Autodesk Inventor part; units mm, degrees
ref_plane "Work Plane1" through (29, 0, 0) normal (0, -1, 0) x (1, 0, 0)
ref_plane "YZ Plane" through (0, 0, 0) normal (1, 0, 0) x (0, 1, 0)
ref_plane "XZ Plane" through (0, 0, 0) normal (0, 1, 0) x (-1, 0, 0)
sketch "Sketch1" plane through (0, 0, 0) normal (0, 0, 1) x (1, 0, 0)
  line L0 (-0.0762, 0) -> (3.175, 0)
  line L1 (3.175, 0) -> (3.175, 1.7526)
  line L2 (3.175, 1.7526) -> (1.5902, 1.7526)
  line L3 (1.5902, 1.7526) -> (0.0001, 1.7526)
  line L4 (0.0001, 1.7526) -> (0, 1.7526)
  line L5 (0, 1.7526) -> (0, 3.3274)
  line L6 (0, 3.3274) -> (-1.8542, 3.3274)
  line L7 (-1.8542, 3.3274) -> (-1.8542, 1.1438)
  line L8 (-1.8542, 1.1438) -> (-0.7366, 1.1438)
  line L9 (-0.7366, 1.1438) -> (-0.0762, 0)
  line L10 (-2.86, 0) -> (4.1808, 0)
  line L11 (0, -0.6655) -> (0, 3.9929)
  line L12 (1.5902, 1.7526) -> (0, 1.7526) construction
  dimension "d1" = 1.5848
  dimension "d2" = 1.5901
  dimension "d3" = 1.8542
  dimension "d4" = 1.1176
  dimension "d5" = 60
  dimension "d6" = 3.5052
  dimension "d7" = 3.5052
  dimension "d8" = 2.2877
  dimension "d9" = 6.6548
  dimension "d26" = 3.175
revolve "Body" add sketch "Sketch1" angle 360 about axis through (-0.0762, 0, 0) along (1, 0, 0)
sketch "Sketch2" plane through (-1.8542, 0, 0) normal (-1, 0, 0) x (0, 0, 1)
  circle A0 centre (0, 0) radius 1.1438
  line L0 (0, -4.6584) -> (0, 4.6584)
  line L1 (-4.6584, 0) -> (4.6584, 0)
  line L2 (1.1438, 0) -> (0.5719, -0.9906)
  line L3 (0.5719, -0.9906) -> (-0.5719, -0.9906)
  line L4 (-0.5719, -0.9906) -> (-1.1438, 0)
  line L5 (-1.1438, 0) -> (-0.5719, 0.9906)
  line L6 (-0.5719, 0.9906) -> (0.5719, 0.9906)
  line L7 (0.5719, 0.9906) -> (1.1438, 0)
extrude "Slot" add sketch "Sketch2" against normal up to next contours L7 A0 | A0 L2 | L6 L0 A0 | A0 L0 L3 | L0 L6 A0 | A0 L3 L0 | L4 A0 | A0 L5
fillet "Fillet1" radius 1.8541 1 edges at (-1.8542, -3.3274, 0)
thread "Thread"
chamfer "Chamfer1" distance 0.4869 distance2 0.4869 1 edges at (3.175, -1.7526, 0) measured on face at (3.175, -0.5672, -0.1398)
ref_plane "Work Plane1" through (29, 0, 0) normal (0, -1, 0) x (1, 0, 0)
fillet "Fillet2" radius 0.1 1 edges at (0.0001, -1.7526, 0)
equation "\"d30\" = R"
equation "\"d17\" = RR"
equation "\"d13\" = GEL"
equation "\"d15\" = -0.5 * SPD + 0.5 * GD"
equation "\"d16\" = GUL"
equation "\"d1\" = GEL"
equation "\"d3\" = KOH"
equation "\"d4\" = INTI"
equation "\"d6\" = GD"
equation "\"d7\" = BDM"
equation "\"d8\" = 1.1547 * SW"
equation "\"d9\" = KOD"
equation "\"d26\" = NLG"
equation "\"GD\" = NND"
equation "\"NLG\" = 3.175"
equation "\"GEL\" = 1.58476"
equation "\"KOD\" = 6.6548"
equation "\"KOH\" = 1.8542"
equation "\"INTI\" = 1.1176"
equation "\"GAL\" = 1.59004"
equation "\"GUL\" = 0.48692"
equation "\"BDM\" = NND"
equation "\"SW\" = 1.9812"
equation "\"RR\" = 1.8541"
equation "\"SPD\" = 2.53136"
equation "\"R\" = 0.1"
equation "\"TOA\" = 30deg"
equation "\"GD1\" = SPD"
equation "\"THREADDIA\" = 3.5052"
equation "\"KOH1\" = 0.381"
equation "\"NND\" = 3.5052"
equation "\"E0\" = 2.28829"
properties part number "ANSI B18.3 - 6 - 32 x 1/8" material "Steel, Mild"
Could you check a few things on this model? Use its own coordinates, in mm. A direction names the side the tool comes from. Coordinates: 2 decimals unless noted, no trailing zeros. Order: outer loops, then holes, each group sorted by start corner. A loop starts at its lowest first (then second) coordinate and runs counter-clockwise, first axis right, second up. Notation, with made-up numbers: (78, 29.5) -> (110, 29.5) arc R13 cw to (110, 53.5) -> close; hole circle Ø11 at (-26, -38). An arc over 180 degrees is marked (long way). One line per item, written item: value. Start each with the question number.
1) If I drill on L1, parallel to Y at x = -0.5, z = -2.5; L2, parallel to Y at x = -1.3, z = 1; L3, parallel to X at y = -1.5, z = -1, over which ranges is the centre line in solid material (lowest first)? Write a range as [from, to].
2) Which directions (+Z, -Z, +X, -X, +Y, -Y) give clear straight access to the entire face, cutting with the end or side of a thin tool? Please do faces 1 (the flat face through (-1.26, -0.502, -0.854)), 2 (the conical face through (0, 1, 2)).
3) We'd pull the mould along Y, two halves only. Please class faces 3 (the flat face through (-1.26, 0.502, 0.854)), 4 (the flat face through (-1, -0.991, 0)), 5 (the flat face through (3.175, 0, 0)), 6 (the cylindrical face through (1.38, 1.67, -0.53)): +Y half, -Y half, draft (parallel to the pull), parting line (faces both ways), or undercut.
4) Imagine slicing it at A-A on x = 1.6. List the corners of the cut face in (y, z) for me.
5) I'm going to push flat-ended pins straight in: pin 1 (1.5 mm diameter, centred on x = 1, y = -1, fed in from +Z); pin 2 (3 mm diameter, centred on x = -1, y = 2.5, fed in from +Z); pin 3 (0.6 mm diameter, centred on x = -1.5, z = 0, fed in from +Y); pin 4 (1 mm diameter, centred on x = 0, z = -0.5, fed in from +Y). Where does each tip first touch, or does it pass through?
Answer list:
1. L1: y = [-2.09, 2.09]
1. L2: y = [-2.61, -0.25], [0.25, 2.61]
1. L3: x = [-1.82, 0.01]
2. face 1: -X
2. face 2: +X
3. face 3: undercut
3. face 4: undercut
3. face 5: draft
3. face 6: parting line
4. outline: circle Ø3.51 at (0, 0)
5. pin 1: stops at z = 1.73
5. pin 2: stops at z = 3.09
5. pin 3: stops at y = 2.89
5. pin 4: stops at y = 3.33
